from build123d import *

# Parameters (mm, degrees)
SKETCH1_W                 = 19.05
SKETCH1_H                 = 19.05
BOSS_EXTRUDE1_DEPTH       = 12.7
SKETCH2_W                 = 25.4
SKETCH2_H                 = 25.4
BOSS_EXTRUDE2_DEPTH       = 12.7
SKETCH3_R                 = 9.525
CUT_EXTRUDE3_DEPTH        = 10.16
TAP_DRILL_FOR_4_40_TAP1_D = 2.2606


with BuildPart() as part:
    # Sketch1 → Boss-Extrude1 (new body)
    with BuildSketch(Plane.XY):
        with Locations((-12.7, 12.7)):
            Rectangle(SKETCH1_W, SKETCH1_H)
    extrude(amount=BOSS_EXTRUDE1_DEPTH)

    # Sketch2 → Boss-Extrude2 (add)
    with BuildSketch(Plane(origin=(0, 0, 0), x_dir=(-1, 0, 0), z_dir=(0, 0, -1))):
        with Locations((12.7, 12.7)):
            Rectangle(SKETCH2_W, SKETCH2_H)
    extrude(amount=BOSS_EXTRUDE2_DEPTH)

    # Sketch3 → Cut-Extrude3 (cut)
    with BuildSketch(Plane(origin=(0, 0, -12.7), x_dir=(-1, 0, 0), z_dir=(0, 0, -1))):
        with Locations((12.7, 12.7)):
            Circle(SKETCH3_R)
    extrude(amount=-CUT_EXTRUDE3_DEPTH, mode=Mode.SUBTRACT)

    # Tap Drill for #4-40 Tap1 (through all)
    with Locations(Plane(origin=(0, 22.225, 0), x_dir=(1, 0, 0), z_dir=(0, 1, 0))):
        with Locations((-9.525, -6.35), (-15.875, -6.35)):
            Hole(TAP_DRILL_FOR_4_40_TAP1_D / 2)


solid = part.part
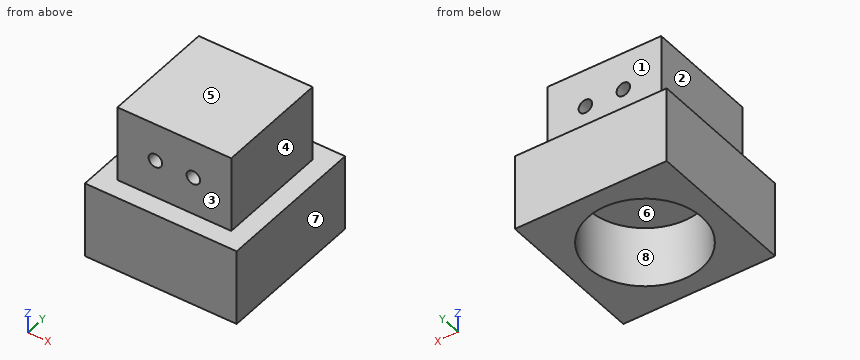
Work out the finished part from the listing and answer in its coordinate system (mm). Face numbers are marked on the shaded views. A direction names the side the tool comes from. Give positions to 0.01 mm unless a question says otherwise; leave off trailing zeros. Write each loop counter-clockwise with the first axis right and the second up, starting at its lowest first coordinate (ties: lowest second). Pieces come first, ordered by that corner, then holes. Notation, with made-up numbers: (71, 54) - (119, 54) arc R16 ccw to (119, 76) - close; hole circle Ø11 at (60.25, 71.5). An arc over 180 degrees is marked (long way). One line per item, written item: value. Start each with the question number.
1. Consider probe 1 along X at (y, z) = (11.25, 6.35) (3 decimals); probe 2 along Y at (x, z) = (-20.25, 8.25) (3 decimals); probe 3 along Z at (x, y) = (-20.75, 10.5). Determine where each line is inside the solid, lowest interval first.
2. Find section D-D (z = -8.25). Write down the section's boundary in (x, y) (3 decimals), then the cut area to 3 significant figures.
3. For a pull along X with two mould halves and no side action, classify the marked faces 5, 6, 7 and 8 as +X half, -X half, draft (parallel to the pull), parting line (faces both ways), or undercut.
4. Find section B-B (y = 12.7). Write down the section's boundary in (x, z) (3 decimals), then the cut area to 3 significant figures.
5. For the marked faces 1, 2, 3 and 4, determine the directions among +Z, -Z, +X, -X, +Y, -Y from which every point of the face is accessible in a straight line to the end or side of a thin tool.
6. Find section C-C (x = -9). Write down the section's boundary in (y, z) (3 decimals), then the cut area to 3 significant figures.
7. Given pin 1 (5 mm diameter, centred on y = 5.5, z = 5, fed in from -X) (3 decimals); pin 2 (5 mm diameter, centred on x = -8.5, z = 7, fed in from +Y) (3 decimals); pin 3 (10 mm diameter, centred on x = -10.5, z = 9.5, fed in from -Y) (3 decimals), each flat-ended and moving along its own axis, determine where each tip first touches the part or whether it passes through.
8. Find section A-A (z = 6.35). Write down the section's boundary in (x, y) (3 decimals).
Geometry results:
1. probe 1: -22.225 to -17.005, -14.745 to -10.655, -8.395 to -3.175
1. probe 2: 3.175 to 22.225
1. probe 3: -2.54 to 12.7
2. outline: (-25.4, 0) - (0, 0) - (0, 25.4) - (-25.4, 25.4) - close; hole circle Ø19.05 at (-12.7, 12.7)
2. area: 360 mm2
3. face 5: draft
3. face 6: undercut
3. face 7: +X half
3. face 8: undercut
4. outline: (-25.4, -12.7) - (-22.225, -12.7) - (-22.225, -2.54) - (-3.175, -2.54) - (-3.175, -12.7) - (0, -12.7) - (0, 0) - (-3.175, 0) - (-3.175, 12.7) - (-22.225, 12.7) - (-22.225, 0) - (-25.4, 0) - close; hole circle Ø2.261 at (-15.875, 6.35); hole circle Ø2.261 at (-9.525, 6.35)
4. area: 363 mm2
5. face 1: +Z, +X, -X, +Y
5. face 2: +Z, -X, +Y, -Y
5. face 3: +Z, +X, -X, -Y
5. face 4: +Z, +X, +Y, -Y
6. outline: (0, -12.7) - (3.923, -12.7) - (3.923, -2.54) - (21.477, -2.54) - (21.477, -12.7) - (25.4, -12.7) - (25.4, 0) - (22.225, 0) - (22.225, 5.349) - (3.175, 5.349) - (3.175, 0) - (0, 0) - close; (3.175, 7.351) - (22.225, 7.351) - (22.225, 12.7) - (3.175, 12.7) - close
6. area: 348 mm2
7. pin 1: x = -22.225
7. pin 2: y = 22.225
7. pin 3: y = 3.175
8. outline: (-22.225, 3.175) - (-17.005, 3.175) - (-17.005, 22.225) - (-22.225, 22.225) - close; (-14.745, 3.175) - (-10.655, 3.175) - (-10.655, 22.225) - (-14.745, 22.225) - close; (-8.395, 3.175) - (-3.175, 3.175) - (-3.175, 22.225) - (-8.395, 22.225) - close
